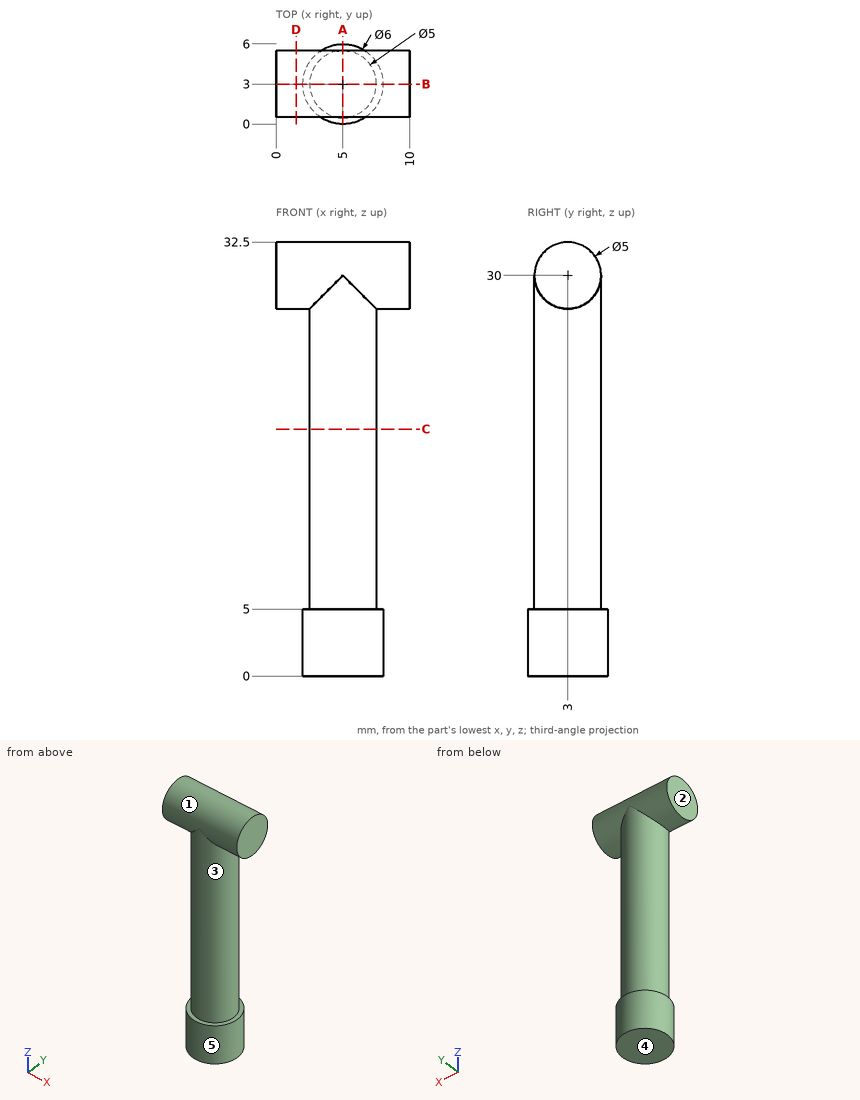
Here's the drawing with two shaded views (mm, measured from the low corner). I have some questions. A direction names the side the tool comes from. Give positions to 0.01 mm unless a question says otherwise; leave off trailing zeros. Write each loop counter-clockwise with the first axis right and the second up, starting at its lowest first coordinate (ties: lowest second). Pieces come first, ordered by that corner, then holes. Notation, with made-up numbers: (58.5, 89.5) -> (71.5, 89.5) arc R12 cw to (71.5, 96.5) -> close; hole circle Ø4 at (17.5, -5.75). An arc over 180 degrees is marked (long way). Use one line per item in the form item = value. Start each with the question number.
1. Imagine slicing it at A-A on x = 5. List the corners of the cut face in (y, z) for me, plus the area to 3 significant figures.
2. If I drill on L1, parallel to Z at x = 7.25, y = 1.1; L2, parallel to X at y = 1.15, z = 16; L3, parallel to Z at x = 9.5, y = 2.1, over which ranges is the centre line in solid material (lowest first)?
3. Will these pins go through, and if not, where does the flat tip stop? pin 1 Ø5 at (x, z) = (7.5, 28.5) entering from -Y; pin 2 Ø2 at (y, z) = (2.5, 9.5) entering from -X; pin 3 Ø1 at (x, z) = (3.5, 26) entering from +Y.
4. Imagine slicing it at C-C on z = 18.5. List the corners of the cut face in (x, y) for me, plus the area to 3 significant figures.
5. Imagine slicing it at D-D on x = 1.5. List the corners of the cut face in (y, z) for me.
6. Thinking about a two-plate mould opening in Z: for the marked faces 3, 4 and 5, which applies, +Z half, -Z half, draft (parallel to the pull), parting line (faces both ways), or undercut?
7. Imagine slicing it at B-B on y = 3. List the corners of the cut face in (x, z) for me, plus the area to 4 significant figures.
8. On a 3-axis mill with a long thin cutter (end or side, diameter ignored), from which of +Z, -Z, +X, -X, +Y, -Y can I reach the whole of each face in a straight line? I mean the marked faces 1 and 2. Say none if no direction works.
Entries:
q1.outline = (0, 0) -> (6, 0) -> (6, 5) -> (5.5, 5) -> (5.5, 30) arc R2.5 ccw to (0.5, 30) -> (0.5, 5) -> (0, 5) -> close
q1.area = 165 mm²
q2.L1 = 0 to 5, 28.38 to 31.62
q2.L2 = 3.32 to 6.68
q2.L3 = 27.67 to 32.33
q3.pin_1 = 0.5
q3.pin_2 = 2.5
q3.pin_3 = 5.29
q4.outline = circle Ø5 at (5, 3)
q4.area = 19.6 mm²
q5.outline = circle Ø5 at (3, 30)
q6.face_3 = undercut
q6.face_4 = -Z half
q6.face_5 = draft
q7.outline = (0, 27.5) -> (2.5, 27.5) -> (2.5, 5) -> (2, 5) -> (2, 0) -> (8, 0) -> (8, 5) -> (7.5, 5) -> (7.5, 27.5) -> (10, 27.5) -> (10, 32.5) -> (0, 32.5) -> close
q7.area = 192.5 mm²
q8.face_1 = none
q8.face_2 = +Z, -Z, -X, +Y, -Y
